Could you check a few things on this drawing? It's one solid part, dimensions in mm from its lowest x, y, z. Give positions to 0.01 mm unless a question says otherwise; leave off trailing zeros. Loops run counter-clockwise (first coordinate to the right, second up) from the corner with the lowest first, then second, coordinate; pieces in that order, holes last. Notation, with made-up numbers: (84.25, 69) - (142.25, 69) arc R21 ccw to (142.25, 80) - close; hole circle Ø5 at (83.25, 57). An arc over 180 degrees is marked (long way). Answer as a JSON object with one key per item and string values.
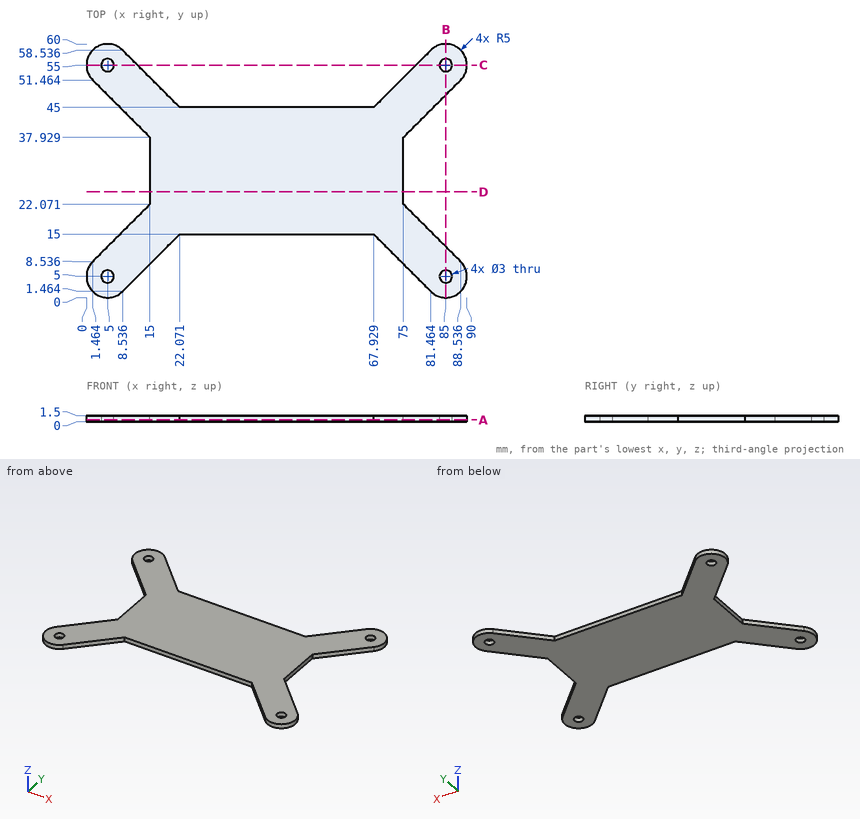
1) I need wall thicknesses on L1, parallel to Y at x = 85, z = 1; L2, parallel to X at y = 36.5, z = 0.7; L3, parallel to X at y = 50.5, z = 0.5. Which ranges of each line are inside material? Lowest first, please.
Check sheet entries:
{"L1": "0 to 3.5, 6.5 to 12.07, 47.93 to 53.5, 56.5 to 60", "L2": "15 to 75", "L3": "2.43 to 16.57, 73.43 to 87.57"}
2) Imagine slicing it at C-C on y = 55. Write out the boundary of the cut face in (x, z).
Check sheet entries:
{"outline": "(0, 0) - (3.5, 0) - (3.5, 1.5) - (0, 1.5) - close; (6.5, 0) - (12.07, 0) - (12.07, 1.5) - (6.5, 1.5) - close; (77.93, 0) - (83.5, 0) - (83.5, 1.5) - (77.93, 1.5) - close; (86.5, 0) - (90, 0) - (90, 1.5) - (86.5, 1.5) - close"}
3) I'm going to push flat-ended pins straight in: P1, Ø0.8, axis at x = 41, z = 0.5, coming from the +Y side; P2, Ø0.8, axis at x = 55.5, z = 1, coming from the -Y side; P3, Ø0.8, axis at y = 31, z = 1, coming from the -X side; P4, Ø2.5, axis at x = 5, y = 55, coming from the +Z side. Where does each tip first touch, or does it pass through?
Check sheet entries:
{"P1": "y = 45", "P2": "y = 15", "P3": "x = 15", "P4": "through"}
4) Imagine slicing it at D-D on y = 25. Write out the boundary of the cut face in (x, z).
Check sheet entries:
{"outline": "(15, 0) - (75, 0) - (75, 1.5) - (15, 1.5) - close"}
5) Imagine slicing it at A-A on z = 0.5. Write out the boundary of the cut face in (x, y) (1 decimal).
Check sheet entries:
{"outline": "(1.5, 8.5) arc R5 ccw to (8.5, 1.5) - (22.1, 15) - (67.9, 15) - (81.5, 1.5) arc R5 ccw to (88.5, 8.5) - (75, 22.1) - (75, 37.9) - (88.5, 51.5) arc R5 ccw to (81.5, 58.5) - (67.9, 45) - (22.1, 45) - (8.5, 58.5) arc R5 ccw to (1.5, 51.5) - (15, 37.9) - (15, 22.1) - close; hole circle Ø3 at (5, 5); hole circle Ø3 at (5, 55); hole circle Ø3 at (85, 5); hole circle Ø3 at (85, 55)"}
6) Imagine slicing it at B-B on x = 85. Write out the boundary of the cut face in (y, z).
Check sheet entries:
{"outline": "(0, 0) - (3.5, 0) - (3.5, 1.5) - (0, 1.5) - close; (6.5, 0) - (12.07, 0) - (12.07, 1.5) - (6.5, 1.5) - close; (47.93, 0) - (53.5, 0) - (53.5, 1.5) - (47.93, 1.5) - close; (56.5, 0) - (60, 0) - (60, 1.5) - (56.5, 1.5) - close"}
